from build123d import *

# Parameters (mm, degrees)
CROQUIS1_R              = 10
SALIENTE_EXTRUIR1_DEPTH = 10
CROQUIS2_R              = 15
CROQUIS2_R_2            = 10
SALIENTE_EXTRUIR2_DEPTH = 35


with BuildPart() as part:
    # Croquis1 → Saliente-Extruir1 (new body)
    with BuildSketch(Plane.XY):
        with BuildLine():
            Line((-49.292513238, 22.5), (90.707486762, 22.5))
            ThreePointArc((90.707486762, 22.5), (105.707486762, 7.5), (90.707486762, -7.5))
            Line((90.707486762, -7.5), (-49.292513238, -7.5))
            ThreePointArc((-49.292513238, -7.5), (-64.292513238, 7.5), (-49.292513238, 22.5))
        make_face()
        with Locations((-49.292513238, 7.5)):
            Circle(CROQUIS1_R, mode=Mode.SUBTRACT)
        with Locations(Location((90.707486762, 7.5, 0), (0, 0, 180))):
            Circle(CROQUIS1_R, mode=Mode.SUBTRACT)
    extrude(amount=SALIENTE_EXTRUIR1_DEPTH)

    # Croquis2 → Saliente-Extruir2 (add)
    with BuildSketch(Plane.XY.offset(10)):
        with Locations(Location((-49.292513238, 7.5, 0), (0, 0, 270))):
            Circle(CROQUIS2_R)
        with Locations((-49.292513238, 7.5)):
            Circle(CROQUIS2_R_2, mode=Mode.SUBTRACT)
    extrude(amount=SALIENTE_EXTRUIR2_DEPTH)


solid = part.part
Here's how the part is built. I have some questions about the finished solid (model axes, mm). A direction names the side the tool comes from. Coordinates: 2 decimals unless noted, no trailing zeros. Loops run counter-clockwise (first coordinate to the right, second up) from the corner with the lowest first, then second, coordinate; pieces in that order, holes last.
1. Imagine slicing it at C-C, the plane y = 20. Please give me the cut outline in (x, z).
2. For faces 4 (the cylindrical face through (-63.936, 10.752, 22.185)), 5 (the flat face through (22, 8, 0)), which set-ups out of +Z, -Z, +X, -X, +Y, -Y let a thin tool reach every point of the face, with its end or its side?
3. Imagine slicing it at D-D, the plane x = -16. Please give me the cut outline in (y, z), and give its area (3 significant figures).
4. I need wall thicknesses on L1, parallel to Z at x = 94, y = -3.5; L2, parallel to X at y = 14.75, z = 42.5; L3, parallel to X at y = 10, z = 3.5. Which ranges of each line are inside material? Lowest first, please.
5. Imagine slicing it at A-A, the plane y = 7.5. Please give me the cut outline in (x, z).
6. If we mould it in two halves opening along Y, with no side actions, what happens to faces 1 (the flat face through (20, 22.5, 5)), 2 (the cylindrical face through (100.7, 7.1, 4.9)), 3 (the flat face through (-52.4, -2.3, 45))? For each: pulls with the +Y half, pulls with the -Y half, needs draft (parallel to the pull), parting line crosses it, or undercut.
7. Imagine slicing it at B-B, the plane z = 32. Please give me the cut outline in (x, y).
8. For P1, Ø8, axis at y = 2, z = 6.5, coming from the -X side; P2, Ø1.5, axis at y = 16.5, z = 12.5, coming from the +X side; P3, Ø4, axis at y = 16.5, z = 15, coming from the +X side; P4, Ø16, axis at x = -49.29, y = 7.5, coming from the -Z side, each with a flat end and sliding along its axis, tell me the tip position at first contact or that it passes through.
Taken from the geometry:
1. outline: (-57.58, 0) - (99, 0) - (99, 10) - (-41, 10) - (-41, 45) - (-57.58, 45) - close
2. face 4: +Z
2. face 5: -Z, +X, -X, +Y, -Y
3. outline: (-7.5, 0) - (22.5, 0) - (22.5, 10) - (-7.5, 10) - close
3. area: 300 mm2
4. L1: z = 0 to 10
4. L2: x = -62.42 to -56.18, -42.41 to -36.16
4. L3: x = -64.08 to -58.97, -39.61 to 81.03, 100.39 to 105.5
5. outline: (-64.29, 0) - (-59.29, 0) - (-59.29, 45) - (-64.29, 45) - close; (-39.29, 0) - (80.71, 0) - (80.71, 10) - (-34.29, 10) - (-34.29, 45) - (-39.29, 45) - close; (100.71, 0) - (105.71, 0) - (105.71, 10) - (100.71, 10) - close
6. face 1: pulls with the +Y half
6. face 2: undercut
6. face 3: needs draft
7. outline: circle Ø30 at (-49.29, 7.5); hole circle Ø20 at (-49.29, 7.5)
8. P1: stops at x = -64.22
8. P2: stops at x = -36.77
8. P3: stops at x = -36.03
8. P4: passes through
